Input: part model. Units: mm. Frame: model coordinates. Face numbers are marked on the shaded views. A direction names the side the tool comes from. Coordinates: 2 decimals unless noted, no trailing zeros. Loops run counter-clockwise (first coordinate to the right, second up) from the corner with the lowest first, then second, coordinate; pieces in that order, holes last.
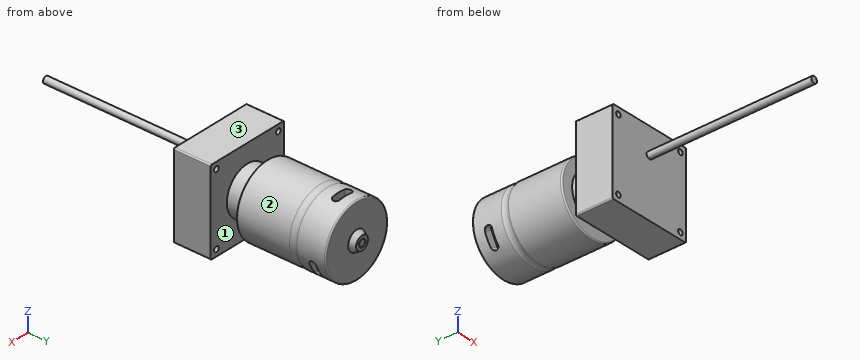
```python
from build123d import *

# Parameters (mm, degrees)
BOSS_EXTRUDE1_DEPTH = 28
SKETCH2_R           = 18
BOSS_EXTRUDE2_DEPTH = 15
SKETCH3_R           = 27
BOSS_EXTRUDE3_DEPTH = 68
FILLET1_R           = 1
FILLET2_R           = 1
SKETCH4_R           = 2
CUT_EXTRUDE1_DEPTH  = 29
SKETCH5_R           = 2.5
BOSS_EXTRUDE4_DEPTH = 125
SKETCH7_R           = 7.5
BOSS_EXTRUDE5_DEPTH = 4
BOSS_EXTRUDE5_TAPER = 30
CUT_EXTRUDE2_DEPTH  = 10
CIRPATTERN1_COUNT   = 3
CUT_EXTRUDE3_DEPTH  = 10
CIRPATTERN2_COUNT   = 3


with BuildPart() as part:
    # Sketch1 → Boss-Extrude1 (new body)
    with BuildSketch(Plane(origin=(0, 0, 0), x_dir=(1, 0, 0), z_dir=(0, 1, 0))):
        with BuildLine():
            Line((-31, 32), (31, 32))
            ThreePointArc((31, 32), (31.707106781, 31.707106781), (32, 31))
            Line((32, 31), (32, -31))
            ThreePointArc((32, -31), (31.707106781, -31.707106781), (31, -32))
            Line((31, -32), (-31, -32))
            ThreePointArc((-31, -32), (-31.707106781, -31.707106781), (-32, -31))
            Line((-32, -31), (-32, 31))
            ThreePointArc((-32, 31), (-31.707106781, 31.707106781), (-31, 32))
        make_face()
    extrude(amount=BOSS_EXTRUDE1_DEPTH)

    # Sketch2 → Boss-Extrude2 (add)
    with BuildSketch(Plane(origin=(0, 28, 0), x_dir=(1, 0, 0), z_dir=(0, 1, 0))):
        Circle(SKETCH2_R)
    extrude(amount=BOSS_EXTRUDE2_DEPTH)

    # Sketch3 → Boss-Extrude3 (add)
    with BuildSketch(Plane(origin=(0, 43, 0), x_dir=(1, 0, 0), z_dir=(0, 1, 0))):
        Circle(SKETCH3_R)
    extrude(amount=BOSS_EXTRUDE3_DEPTH)

    # Fillet1
    fillet1_edges = [part.edges().sort_by_distance(p)[0] for p in [
        (-27, 43, 0),
    ]]
    fillet(fillet1_edges, radius=FILLET1_R)

    # Fillet2
    fillet2_edges = [part.edges().sort_by_distance(p)[0] for p in [
        (-27, 111, 0),
    ]]
    fillet(fillet2_edges, radius=FILLET2_R)

    # Sketch4 → Cut-Extrude1 (cut, through all)
    with BuildSketch(Plane(origin=(0, 28, 0), x_dir=(1, 0, 0), z_dir=(0, 1, 0))):
        with Locations((-27, 27)):
            Circle(SKETCH4_R)
        with Locations((27, 27)):
            Circle(SKETCH4_R)
        with Locations((27, -27)):
            Circle(SKETCH4_R)
        with Locations((-27, -27)):
            Circle(SKETCH4_R)
    extrude(amount=-CUT_EXTRUDE1_DEPTH, mode=Mode.SUBTRACT)

    # Sketch5 → Boss-Extrude4 (add)
    with BuildSketch(Plane.XZ):
        with Locations((0, 12)):
            Circle(SKETCH5_R)
    extrude(amount=BOSS_EXTRUDE4_DEPTH)

    # Sketch6 → Cut-Revolve1 (revolve, cut)
    with BuildSketch(Plane(origin=(0, 0, 0), x_dir=(0, 0, -1), z_dir=(1, 0, 0))):
        with BuildLine():
            Line((27, 88.942293347), (27, 83.446507899))
            ThreePointArc((27, 83.446507899), (26.371517202, 86.194400623), (27, 88.942293347))
        make_face()
    revolve(axis=Axis((0, 111, 0), (0, -1, 0)), mode=Mode.SUBTRACT)

    # Sketch7 → Boss-Extrude5 (add)
    with BuildSketch(Plane(origin=(0, 111, 0), x_dir=(1, 0, 0), z_dir=(0, 1, 0))):
        Circle(SKETCH7_R)
    extrude(amount=BOSS_EXTRUDE5_DEPTH, taper=BOSS_EXTRUDE5_TAPER)

    # Sketch8 → Cut-Extrude2 (cut)
    with BuildSketch(Plane.XY.offset(30)):
        with BuildLine():
            Line((-5.065984647, 102.694191022), (4.934015353, 102.694191022))
            ThreePointArc((4.934015353, 102.694191022), (7.628206376, 100), (4.934015353, 97.305808978))
            Line((4.934015353, 97.305808978), (-5.065984647, 97.305808978))
            ThreePointArc((-5.065984647, 97.305808978), (-7.760175669, 100), (-5.065984647, 102.694191022))
        make_face()
    cut_extrude2 = extrude(amount=-CUT_EXTRUDE2_DEPTH, mode=Mode.SUBTRACT)

    # CirPattern1: Cut-Extrude2 ×3 about axis
    cirpattern1_axis = Axis((0, 0, 0), (0, 1, 0))
    for i in range(1, CIRPATTERN1_COUNT):
        add(cut_extrude2.rotate(cirpattern1_axis, i * 360 / CIRPATTERN1_COUNT), mode=Mode.SUBTRACT)

    # Sketch9 → Cut-Extrude3 (cut)
    with BuildSketch(Plane(origin=(0, 115, 0), x_dir=(1, 0, 0), z_dir=(0, 1, 0))):
        with BuildLine():
            ThreePointArc((2.424806001, 1.617896807), (0.319254394, 2.897473184), (-2.014380463, 2.107022917))
            ThreePointArc((-2.014380463, 2.107022917), (-2.021480856, 1.791146289), (-1.705604229, 1.784045896))
            ThreePointArc((-1.705604229, 1.784045896), (0.270317179, 2.453331239), (2.053117296, 1.36989595))
            ThreePointArc((2.053117296, 1.36989595), (2.362962077, 1.308052026), (2.424806001, 1.617896807))
        make_face()
    cut_extrude3 = extrude(amount=-CUT_EXTRUDE3_DEPTH, mode=Mode.SUBTRACT)

    # CirPattern2: Cut-Extrude3 ×3 about axis
    cirpattern2_axis = Axis((0, 0, 0), (0, 1, 0))
    for i in range(1, CIRPATTERN2_COUNT):
        add(cut_extrude3.rotate(cirpattern2_axis, i * 360 / CIRPATTERN2_COUNT), mode=Mode.SUBTRACT)


solid = part.part
```
Item 1: Section query A-A (y = 100). Output: boundary loops of the cut face in (x, z).
Result:
outline: (-26.24, -6.34) - (-21.13, -3.39) - (-13.44, -16.72) - (-18.52, -19.65) arc R27 ccw to (18.62, -19.56) - (13.51, -16.61) - (21.2, -3.28) - (26.28, -6.21) arc R27 ccw to (7.63, 25.9) - (7.63, 20) - (-7.76, 20) - (-7.76, 25.86) arc R27 ccw to start
Item 2: Line query: L1, parallel to Z at x = -27, y = 11; L2, parallel to Y at x = -18, z = -10. Output: solid intervals per line, ascending.
Result:
L1: z = -32 to -29, -25 to 25, 29 to 32
L2: y = 0 to 28, 43 to 97.31, 102.69 to 111
Item 3: Section query C-C (y = 36.5). Output: boundary loops of the cut face in (x, z).
Result:
outline: circle Ø36 at (0, 0)
Item 4: Reachability of the marked faces 1, 2 and 3 from +Z, -Z, +X, -X, +Y, -Y: full face, straight path, thin tool, end or side. Return the list, or none.
Result:
face 1: none
face 2: +Y
face 3: +Z, +X, -X, +Y, -Y
Item 5: Section query B-B (y = -11). Output: boundary loops of the cut face in (x, z), then the cut area to 3 significant figures.
Result:
outline: circle Ø5 at (0, 12)
area: 19.6 mm2
Item 6: Contact query for flat-ended pins moving along their axis: P1, Ø4.5, axis at x = 2.5, y = 99.5, coming from the +Z side; P2, Ø1, axis at x = 6, z = 14.5, coming from the -Y side; P3, Ø3, axis at x = -10, z = -2, coming from the +Y side; P4, Ø3, axis at x = -27, z = 27, coming from the -Y side. Output: stop coordinate, or through.
Result:
P1: stops at z = 26.93
P2: stops at y = 0
P3: stops at y = 111
P4: passes through
